from build123d import *

# Parameters (mm, degrees)
F1_DEPTH = 9.5
F2_R     = 2
F3_DEPTH = 9.001
F5_R     = 3.75
F6_DEPTH = 5


with BuildPart() as f1:
    # F0 (on Right) → F1 (new body)
    with BuildSketch(Plane.YZ):
        with BuildLine():
            Line((1.232946, 1), (9.949874, 1))
            ThreePointArc((9.949874, 1), (0, 10), (-9.949874, 1))
            Line((-9.949874, 1), (-1.232946, 1))
            ThreePointArc((-1.232946, 1), (0, 1.5875), (1.232946, 1))
        make_face()
    extrude(amount=F1_DEPTH)

    # F2 (on face) → F3 (cut, through all)
    with BuildSketch(Plane(origin=(0, 0, 1), x_dir=(1, 0, 0), z_dir=(0, 0, -1))):
        with Locations((4.25, 6.5)):
            Circle(F2_R)
        with Locations((4.25, -6.5)):
            Circle(F2_R)
    extrude(amount=-F3_DEPTH, mode=Mode.SUBTRACT)

    # F5 (on offset) → F6 (cut)
    with BuildSketch(Plane.XY.offset(10)):
        with Locations((4.25, 6.5)):
            Circle(F5_R)
    extrude(amount=-F6_DEPTH, mode=Mode.SUBTRACT)


solid = f1.part
Could you check a few things on this model? Use its own coordinates, in mm. A direction names the side the tool comes from. Give positions to 0.01 mm unless a question says otherwise; leave off trailing zeros. Order: outer loops, then holes, each group sorted by start corner. A loop starts at its lowest first (then second) coordinate and runs counter-clockwise, first axis right, second up. Notation, with made-up numbers: (38, -18) - (76, -18) arc R26 ccw to (76, 4) - close; hole circle Ø3 at (-7.75, 13). An arc over 180 degrees is marked (long way). Return JSON: item names as keys, results as strings. Group by question number.
Q1. Thinking about a two-plate mould opening in X: for faces 1 (the face through (4, 4, 5)), 2 (the face through (9.5, 0, 5)), 3 (the face through (0, 0, 5)), 4 (the face through (6, 5, 1)), which applies, pulls with the +X half, pulls with the -X half, needs draft (parallel to the pull), parting line crosses it, or undercut?
Q2. Suppose I cut it at B-B, the plane x = 2.5. Please give me the cut outline in (y, z) (1 decimal).
Q3. Which directions (+Z, -Z, +X, -X, +Y, -Y) give clear straight access to the entire face, cutting with the end or side of a thin tool? Please do faces 5 (the face through (4.14, 2.75, 6.83)), 6 (the face through (6, -5, 1)).
Q4. Will these pins go through, and if not, where does the flat tip stop? pin 1 Ø1 at (x, y) = (8, 1) entering from -Z; pin 2 Ø4.5 at (x, y) = (5, 6) entering from +Z; pin 3 Ø4.5 at (x, y) = (4.25, -6.5) entering from +Z; pin 4 Ø4 at (x, z) = (7, 7.5) entering from -Y.
Q5. Suppose I cut it at D-D, the plane z = 4. Please give me the cut outline in (x, y), and give its area (3 significant figures).
Q6. Please list where these lines run through material, in increasing order: line 1 along X through (y, z) = (6.5, 2.35); line 2 along Y through (x, z) = (4.25, 2.8); line 3 along Z through (x, y) = (9, 2.75). Write a range as [from, to].
Q7. Suppose I cut it at C-C, the plane z = 7. Please give me the cut outline in (x, y), and give its area (3 significant figures).
Q8. Suppose I cut it at A-A, the plane y = -6. Please give me the cut outline in (x, z).
Resolved:
{
 "1": {"face 1": "undercut", "face 2": "pulls with the +X half", "face 3": "pulls with the -X half", "face 4": "needs draft"},
 "2": {"outline": "(-9.9, 1) - (-7.5, 1) - (-7.5, 6.7) arc R10 ccw to start; (-5.5, 1) - (-1.2, 1) arc R1.6 cw to (1.2, 1) - (5.5, 1) - (5.5, 5) - (3.2, 5) - (3.2, 9.5) arc R10 ccw to (-5.5, 8.3) - close; (7.5, 1) - (9.9, 1) arc R10 ccw to (8.7, 5) - (7.5, 5) - close"},
 "3": {"face 5": "+Z", "face 6": "-Z, +X, -X, +Y, -Y"},
 "4": {"pin 1": "stops at z = 1", "pin 2": "stops at z = 5", "pin 3": "stops at z = 9.05", "pin 4": "stops at y = -8.35"},
 "5": {"outline": "(0, -9.17) - (9.5, -9.17) - (9.5, 9.17) - (0, 9.17) - close; hole circle Ø4 at (4.25, -6.5); hole circle Ø4 at (4.25, 6.5)", "area": "149 mm2"},
 "6": {"line 1": "x = [0, 2.25], [6.25, 9.5]", "line 2": "y = [-9.6, -8.5], [-4.5, 4.5], [8.5, 9.6]", "line 3": "z = [1, 9.61]"},
 "7": {"outline": "(0, -7.14) - (2.36, -7.14) arc R2 cw (long way) to (6.14, -7.14) - (9.5, -7.14) - (9.5, 7.14) - (7.94, 7.14) arc R3.75 cw (long way) to (0.56, 7.14) - (0, 7.14) - close", "area": "100 mm2"},
 "8": {"outline": "(0, 1) - (2.31, 1) - (2.31, 8) - (0, 8) - close; (6.19, 1) - (9.5, 1) - (9.5, 8) - (6.19, 8) - close"}
}
